Source: CAD feature listing. Evaluate the final solid. Frame: model axes, mm. A direction names the side the tool comes from. Round coordinates to 2 decimals unless told otherwise and drop trailing zeros. Loops run counter-clockwise (first coordinate to the right, second up) from the corner with the lowest first, then second, coordinate; pieces in that order, holes last.
Item 1: First-contact query: P1, Ø6, axis at x = 80, y = 7, coming from the -Z side; P2, Ø8, axis at x = 28, y = 8, coming from the +Z side; P3, Ø6, axis at x = 101, y = -1.5, coming from the +Z side. Flat tips, straight axial feed; report the tip coordinate or a pass-through.
Item 2: Access query for faces 1 (the cylindrical face through (-2.75, -12.4, 572.92)), 2 (the cylindrical face through (113.714, 3.815, 387.883)). Directions: +Z, -Z, +X, -X, +Y, -Y. A direction counts if a zero-diameter tool reaches every point of the face in a straight line with its end or side. Return the directions, or none.
Item 3: Ray query, L1, parallel to Z at x = 34, y = -1.5; L2, parallel to X at y = 1.5, z = 471; L3, parallel to Y at x = -0.5, z = 262. Return the intervals inside material, ascending.
Item 4: Section query A-A on x = 46. Return loops of the section in (y, z).
Item 5: Section query C-C on z = 139. Return loops of the section in (x, y), then the cut area to 3 significant figures.
Item 6: Pull-direction query (Z, two-part tool) for faces 3 (the flat face through (0, 0, 673.1)), 4 (the cylindrical face through (-2.75, -12.4, 154.53)), 5 (the flat face through (0, 0, 0)), 6 (the cylindrical face through (54.375, 3.815, 318.086)); classes: released by +Z, released by -Z, zero draft, split by the parting line, or undercut.
Item 7: Section query B-B on y = 5. Return loops of the section in (x, z).
```python
from build123d import *

# Parameters (mm, degrees)
F1_R = 12.7


with BuildPart() as f2:
    # F2: sweep along a path in F0
    with BuildLine(Plane.XZ) as f2_path:
        Line((0, 0), (0, 304.8))
        ThreePointArc((0, 304.8), (7.4394877579, 322.7605122421), (25.4, 330.2))
        Line((25.4, 330.2), (82.55, 330.2))
        ThreePointArc((82.55, 330.2), (96.0203841816, 335.7796158184), (101.6, 349.25))
        Line((101.6, 349.25), (101.6, 425.45))
        ThreePointArc((101.6, 425.45), (96.0203841816, 438.9203841816), (82.55, 444.5))
        Line((82.55, 444.5), (25.4, 444.5))
        ThreePointArc((25.4, 444.5), (7.4394877579, 451.9394877579), (0, 469.9))
        Line((0, 469.9), (0, 673.1))
    # F1 (on Top) → F2 (sweep)
    with BuildSketch(Plane.XY):
        Circle(F1_R)
    sweep(path=f2_path.line)


solid = f2.part
```
Data:
1. P1: stops at z = 318.15
1. P2: stops at z = 456.55
1. P3: stops at z = 453.12
2. face 1: +Z
2. face 2: none
3. L1: z = 317.59 to 342.81, 431.89 to 457.11
3. L2: x = -12.61 to 12.61
3. L3: y = -12.69 to 12.69
4. outline: circle Ø25.4 at (0, 330.2); circle Ø25.4 at (0, 444.5)
5. outline: circle Ø25.4 at (0, 0)
5. area: 507 mm2
6. face 3: released by +Z
6. face 4: zero draft
6. face 5: released by -Z
6. face 6: undercut
7. outline: (-11.67, 0) - (11.67, 0) - (11.67, 304.8) arc R13.73 cw to (25.4, 318.53) - (82.55, 318.53) arc R30.72 ccw to (113.27, 349.25) - (113.27, 425.45) arc R30.72 ccw to (82.55, 456.17) - (25.4, 456.17) arc R13.73 cw to (11.67, 469.9) - (11.67, 673.1) - (-11.67, 673.1) - (-11.67, 469.9) arc R37.07 ccw to (25.4, 432.83) - (82.55, 432.83) arc R7.38 cw to (89.93, 425.45) - (89.93, 349.25) arc R7.38 cw to (82.55, 341.87) - (25.4, 341.87) arc R37.07 ccw to (-11.67, 304.8) - close
